Check sheet for the modelled part. Datum: model origin and axes. Units: mm. A direction names the side the tool comes from. Coordinates: 2 decimals unless noted, no trailing zeros. Write each loop counter-clockwise with the first axis right and the second up, starting at its lowest first coordinate (ties: lowest second). Pieces come first, ordered by that corner, then holes. Notation, with made-up numbers: (63.5, -15) - (74.5, -15) arc R9 cw to (74.5, -11) - close; hole circle Ø7 at (-39.5, 42.25). An arc over 180 degrees is marked (long way). Write each question's results on one line, items separated by ' | '.
from build123d import *

# Parameters (mm, degrees)
SKETCH1_W                 = 114.3
SKETCH1_H                 = 177.8
SKETCH1_W_2               = 101.6
SKETCH1_H_2               = 165.1
BOSS_EXTRUDE1_DEPTH       = 4.7625
SKETCH2_W                 = 12.38677804
SKETCH2_H                 = 4.7625
SKETCH2_W_2               = 12.7
BOSS_EXTRUDE2_DEPTH       = 4.7625
SKETCH3_W                 = 12.7
SKETCH3_H                 = 4.7625
BOSS_EXTRUDE3_DEPTH       = 4.7625
FILLET1_R                 = 2.54
SKETCH4_W                 = 101.6
SKETCH4_H                 = 6.35
SKETCH4_W_2               = 114.3
BOSS_EXTRUDE4_DEPTH       = 4.7625
FILLET2_R                 = 2.54
F_6_CLEARANCE_HOLE1_D     = 3.7973
F_6_CLEARANCE_HOLE1_DEPTH = 25.4
F_6_CLEARANCE_HOLE1_TIP   = 1.140824014


with BuildPart() as part:
    # Sketch1 → Boss-Extrude1 (new body)
    with BuildSketch(Plane(origin=(0, 0, 0), x_dir=(1, 0, 0), z_dir=(0, 1, 0))):
        Rectangle(SKETCH1_W, SKETCH1_H)
        Rectangle(SKETCH1_W_2, SKETCH1_H_2, mode=Mode.SUBTRACT)
    extrude(amount=BOSS_EXTRUDE1_DEPTH)

    # Sketch2 → Boss-Extrude2 (add)
    with BuildSketch(Plane.XY.offset(88.9)):
        with Locations((-38.1, 2.38125)):
            Rectangle(SKETCH2_W, SKETCH2_H)
        with Locations((12.7, 2.38125)):
            Rectangle(SKETCH2_W_2, SKETCH2_H)
    extrude(amount=BOSS_EXTRUDE2_DEPTH)

    # Sketch3 → Boss-Extrude3 (add)
    with BuildSketch(Plane(origin=(0, 0, -88.9), x_dir=(-1, 0, 0), z_dir=(0, 0, -1))):
        with Locations((-38.1, 2.38125)):
            Rectangle(SKETCH3_W, SKETCH3_H)
        with Locations((12.7, 2.38125)):
            Rectangle(SKETCH3_W, SKETCH3_H)
    extrude(amount=BOSS_EXTRUDE3_DEPTH)

    # Fillet1
    fillet1_edges = [part.edges().sort_by_distance(p)[0] for p in [
        (50.8, 2.38125, 82.55),
        (50.8, 2.38125, -82.55),
        (-50.8, 2.38125, -82.55),
        (-50.8, 2.38125, 82.55),
    ]]
    fillet(fillet1_edges, radius=FILLET1_R)

    # Sketch4 → Boss-Extrude4 (add)
    with BuildSketch(Plane(origin=(0, 4.7625, 0), x_dir=(1, 0, 0), z_dir=(0, 1, 0))):
        with Locations((0, 9.525)):
            Rectangle(SKETCH4_W, SKETCH4_H)
        with Locations((0, -9.525)):
            Rectangle(SKETCH4_W_2, SKETCH4_H)
    extrude(amount=-BOSS_EXTRUDE4_DEPTH)

    # Fillet2
    fillet2_edges = [part.edges().sort_by_distance(p)[0] for p in [
        (-50.8, 2.38125, -6.35),
        (-50.8, 2.38125, -12.7),
        (50.8, 2.38125, -12.7),
        (50.8, 2.38125, -6.35),
        (-50.8, 2.38125, 12.7),
        (-50.8, 2.38125, 6.35),
        (50.8, 2.38125, 6.35),
        (50.8, 2.38125, 12.7),
    ]]
    fillet(fillet2_edges, radius=FILLET2_R)

    # #6 Clearance Hole1
    with Locations(Plane(origin=(0, 4.7625, 0), x_dir=(-1, 0, 0), z_dir=(0, 1, 0))):
        with Locations((25.4, -9.525), (25.4, 9.525), (-25.4, 9.525), (-25.4, -9.525)):
            Hole(F_6_CLEARANCE_HOLE1_D / 2, depth=F_6_CLEARANCE_HOLE1_DEPTH)
            with Locations((0, 0, -(F_6_CLEARANCE_HOLE1_DEPTH + F_6_CLEARANCE_HOLE1_TIP / 2))):  # 118° drill point
                Cone(0, F_6_CLEARANCE_HOLE1_D / 2, F_6_CLEARANCE_HOLE1_TIP, mode=Mode.SUBTRACT)


solid = part.part
1. Go/stop test with flat-tipped pins: pin 1 (5 mm diameter, centred on x = 25.4, z = -9.525, fed in from +Y); pin 2 (2.5 mm diameter, centred on x = 47.5, y = 1.5, fed in from +Z); pin 3 (1.4 mm diameter, centred on x = -29, y = 2, fed in from -Z); pin 4 (2.5 mm diameter, centred on y = 2, z = -90.5, fed in from -X). Record where each tip stops, or that it passes through.
Values follow:
pin 1: stops at y = 4.76 | pin 2: stops at z = 88.9 | pin 3: stops at z = -88.9 | pin 4: stops at x = -19.05
2. Sectioned sample at C-C (x = -34). Record the cut outline in (y, z), then the cut area to 3 significant figures.
Values follow:
outline: (0, -88.9) - (4.76, -88.9) - (4.76, -82.55) - (0, -82.55) - close; (0, -12.7) - (4.76, -12.7) - (4.76, -6.35) - (0, -6.35) - close; (0, 6.35) - (4.76, 6.35) - (4.76, 12.7) - (0, 12.7) - close; (0, 82.55) - (4.76, 82.55) - (4.76, 93.66) - (0, 93.66) - close | area: 144 mm^2
3. Sectioned sample at B-B (z = 74). Record the cut outline in (x, y), then the cut area to 3 significant figures.
Values follow:
outline: (-57.15, 0) - (-50.8, 0) - (-50.8, 4.76) - (-57.15, 4.76) - close; (50.8, 0) - (57.15, 0) - (57.15, 4.76) - (50.8, 4.76) - close | area: 60.5 mm^2
4. Access from +Z, -Z, +X, -X, +Y, -Y to the whole of each face (thin tool, end or side, straight path). Record for faces 5 (the flat face through (-50.8, 2, 48)), 6 (the flat face through (51, 2, -88.9)), 7 (the flat face through (-6.35, 2, -91)).
Values follow:
face 5: +Y, -Y | face 6: -Z, +X, +Y, -Y | face 7: -Z, +Y, -Y
5. Sectioned sample at D-D (y = 2.7). Give the number of separate pieces and of enclosed holes in the cut face, then the cut area to 3 significant figures.
Values follow:
separate pieces: 1 | enclosed holes: 7 | area: 5,050 mm^2
6. Draft check along X on faces 1 (the flat face through (-51, 2, 88.9)), 2 (the flat face through (44.45, 2, -91)), 3 (the flat face through (-44.293, 2, 91)), 4 (the cylindrical face through (24.99, 2.35, -11.38)). Enter one of: pulls with the +X half, pulls with the -X half, needs draft (parallel to the pull), parting line crosses it, or undercut.
Values follow:
face 1: needs draft | face 2: pulls with the +X half | face 3: pulls with the -X half | face 4: undercut
7. Sectioned sample at A-A (x = 25.4). Record the cut outline in (y, z), then the cut area to 3 significant figures.
Values follow:
outline: (0, -88.9) - (4.76, -88.9) - (4.76, -82.55) - (0, -82.55) - close; (0, -12.7) - (4.76, -12.7) - (4.76, -11.42) - (0, -11.42) - close; (0, -7.63) - (4.76, -7.63) - (4.76, -6.35) - (0, -6.35) - close; (0, 6.35) - (4.76, 6.35) - (4.76, 7.63) - (0, 7.63) - close; (0, 11.42) - (4.76, 11.42) - (4.76, 12.7) - (0, 12.7) - close; (0, 82.55) - (4.76, 82.55) - (4.76, 88.9) - (0, 88.9) - close | area: 84.8 mm^2
8. Material ranges on L1, parallel to Z at x = -39.5, y = 3.35; L2, parallel to Z at x = -25.4, y = 3.5; L3, parallel to Z at x = -11, y = 2.35, recorded low to high. Write a range as [from, to].
Values follow:
L1: z = [-88.9, -82.55], [-12.7, -6.35], [6.35, 12.7], [82.55, 93.66] | L2: z = [-88.9, -82.55], [-12.7, -11.42], [-7.63, -6.35], [6.35, 7.63], [11.42, 12.7], [82.55, 88.9] | L3: z = [-93.66, -82.55], [-12.7, -6.35], [6.35, 12.7], [82.55, 88.9]
